The listing builds one solid part. Answer for the finished solid, in the listing's coordinates (mm). Face numbers are marked on the shaded views. A direction names the side the tool comes from. Round coordinates to 2 decimals unless told otherwise and drop trailing zeros. Loops run counter-clockwise (first coordinate to the right, second up) from the corner with the lowest first, then second, coordinate; pieces in that order, holes last. Notation, with made-up numbers: M -2,17 L 18,17 A16 ccw 18,35 Z; hole C 23,74.25 d3. An arc over 180 degrees is marked long. Put each result on its own line as item: value. Start each with the question number.
(1) Section A-A, the plane y = 17.5 is taken. Determine the outline of the cut face in (x, z).
(2) Flat-ended cylindrical pins translate along their axes: P1, Ø1, axis at x = -17, y = -11, coming from the +Z side; P2, Ø22.5, axis at x = -25, y = -10, coming from the -Z side; P3, Ø13.5, axis at x = -23.5, y = 5.5, coming from the +Z side; P4, Ø7, axis at x = 20.5, z = 4, coming from the +Y side (3 decimals). Find the tip coordinate at first contact, or state that the pin passes through.
(3) Section D-D, the plane x = 68 is taken. Determine the outline of the cut face in (y, z) (3 decimals), then the cut area to 3 significant figures.
(4) Straight lines are drawn through the part: line 1 (X direction, y = -18, z = -1); line 2 (Z direction, x = -71, y = -17); line 3 (Z direction, x = 7.5, y = -20). For each, find the intervals that lie inside material, in ascending order.
(5) Section B-B, the plane y = -14 is taken. Determine the outline of the cut face in (x, z).
(6) Which of the six approach directions +Z, -Z, +X, -X, +Y, -Y give full straight-line access (tool end or side, diameter ignored) to the marked faces 1 and 2?
```python
from build123d import *

# Parameters (mm, degrees)
F0_W     = 292.1
F0_H     = 44.45
F1_DEPTH = 6.35
F2_W     = 130.175
F2_H     = 24.13
F3_DEPTH = 6.351
F4_W     = 80.9625
F4_H     = 44.45
F5_DEPTH = 4.318
F7_DEPTH = 44.45


with BuildPart() as f1:
    # F0 (on Top) → F1 (new body)
    with BuildSketch(Plane.XY):
        Rectangle(F0_W, F0_H)
    extrude(amount=F1_DEPTH)

    # F2 (on face) → F3 (cut, through all)
    with BuildSketch(Plane.XY.offset(6.35)):
        with Locations((0, 10.16)):
            Rectangle(F2_W, F2_H)
    extrude(amount=-F3_DEPTH, mode=Mode.SUBTRACT)

    # F4 (on face) → F5 (join)
    with BuildSketch(Plane(origin=(0, 0, 0), x_dir=(1, 0, 0), z_dir=(0, 0, -1))):
        with Locations((-105.56875, 0)):
            Rectangle(F4_W, F4_H)
        with Locations((105.56875, 0)):
            Rectangle(F4_W, F4_H)
    extrude(amount=F5_DEPTH)

    # F6 (on face) → F7 (join, through all)
    with BuildSketch(Plane.XZ.offset(22.225)):
        Polygon((-146.05, 11.557), (-146.05, 6.35), (-72.7075, 6.35), (-72.7075, 7.713282), align=None)
        Polygon((72.7075, 7.713282), (72.7075, 6.35), (146.05, 6.35), (146.05, 11.557), align=None)
    extrude(amount=-F7_DEPTH)


solid = f1.part
```
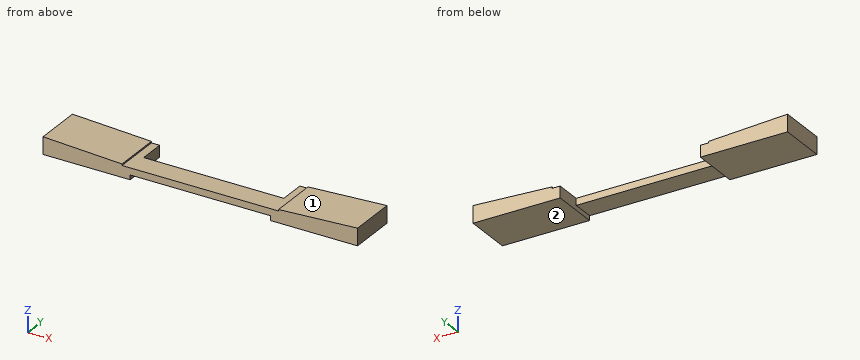
Recorded:
1. outline: M -146.05,-4.32 L -65.09,-4.32 L -65.09,6.35 L -72.71,6.35 L -72.71,7.71 L -146.05,11.56 Z; M 65.09,-4.32 L 146.05,-4.32 L 146.05,11.56 L 72.71,7.71 L 72.71,6.35 L 65.09,6.35 Z
2. P1: stops at z = 6.35
2. P2: stops at z = 0
2. P3: passes through
2. P4: stops at y = -1.905
3. outline: M -22.225,-4.318 L 22.225,-4.318 L 22.225,6.35 L -22.225,6.35 Z
3. area: 474 mm²
4. line 1: x = -146.05 to -65.09, 65.09 to 146.05
4. line 2: z = -4.32 to 6.35
4. line 3: z = 0 to 6.35
5. outline: M -146.05,-4.32 L -65.09,-4.32 L -65.09,0 L 65.09,0 L 65.09,-4.32 L 146.05,-4.32 L 146.05,11.56 L 72.71,7.71 L 72.71,6.35 L -72.71,6.35 L -72.71,7.71 L -146.05,11.56 Z
6. face 1: +Z, +Y, -Y
6. face 2: -Z, +X, -X, +Y, -Y
